Solid Edge part; units mm, degrees
sketch "Sketch1" plane through (0, 0, 0) normal (0, 0, 1) x (1, 0, 0)
  line L0 (-74.7428, -5) -> (-74.7428, -88.7121)
  arc A0 (-70.7682, -93.6058) -> (-74.7428, -88.7121) centre (-69.7428, -88.7121) cw
  arc A1 (-70.7682, -93.6058) -> (70.7677, -93.5993) centre (-0.0157, 244.0613) ccw
  arc A2 (74.7418, -88.7058) -> (70.7677, -93.5994) centre (69.7418, -88.7058) cw
  line L1 (74.7418, -88.7058) -> (74.7418, -5)
  arc A3 (69.7418, 0) -> (74.7418, -5) centre (69.7418, -5) cw
  line L2 (69.7418, 0) -> (65.2418, 0)
  arc A4 (60.2418, -5) -> (65.2418, 0) centre (65.2418, -5) cw
  line L3 (60.2418, -73.162) -> (60.2418, -5)
  arc A5 (56.0999, -78.0878) -> (60.2418, -73.162) centre (55.2418, -73.162) ccw
  arc A6 (-56.1003, -78.0932) -> (56.0999, -78.0878) centre (-0.0157, 244.0613) ccw
  arc A7 (-60.2428, -73.1673) -> (-56.1003, -78.0932) centre (-55.2428, -73.1673) ccw
  line L4 (-60.2428, -73.1673) -> (-60.2428, -5)
  arc A8 (-65.2428, 0) -> (-60.2428, -5) centre (-65.2428, -5) cw
  line L5 (-65.2428, 0) -> (-69.7428, 0)
  arc A9 (-74.7428, -5) -> (-69.7428, 0) centre (-69.7428, -5) cw
extrude "Protrusion1" add sketch "Sketch1" along normal mid plane 12
properties part number "2003-004" material "Plastic"
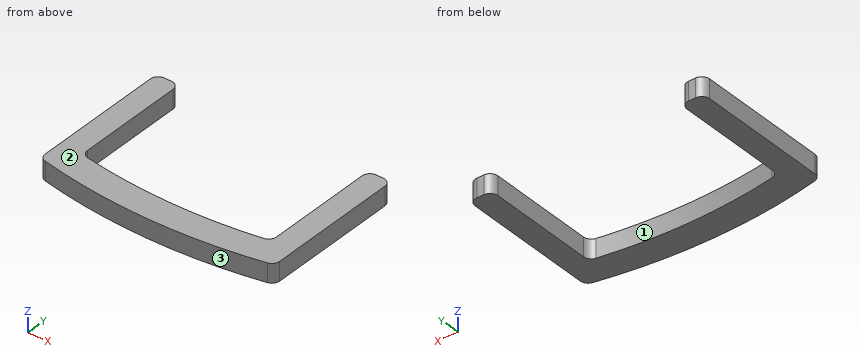
Model file for the job. Use its own axes, mm. Face numbers are marked on the shaded views. Give positions to 0.01 mm unless a question says otherwise; leave off trailing zeros. Write each loop counter-clockwise with the first axis right and the second up, starting at its lowest first coordinate (ties: lowest second). Pieces come first, ordered by that corner, then holes. Notation, with made-up numbers: (-16, 5) - (40, 5) arc R17 cw to (40, 10) - close; hole circle Ø11 at (89, 44). An arc over 180 degrees is marked (long way). One line per question, with ' | ' between items. Start each with the question number.
(1) Wall check: line 1 along X through (y, z) = (-9, 1); line 2 along Y through (x, z) = (3.5, 5.25); line 3 along Y through (x, z) = (55.5, 1.25). Give the ranges that are in metal, low to high. Write a range as from..to.
(2) Pin check, flat tip, straight feed: P1, Ø2, axis at x = -48.5, z = 3.5, coming from the -Y side. Stop position of the tip, or through.
(3) Slice it at A-A on y = -66.5. Write the cut outline in (x, z).
(4) Slice it at B-B on z = 1.5. Write the cut outline in (x, y), plus the area to 3 significant figures.
(5) Slice it at D-D on x = 18.5. Write the cut outline in (y, z), plus the area to 3 significant figures.
(6) Slice it at C-C on x = -20. Write the cut outline in (y, z), plus the area to 3 significant figures.
(7) Two-plate mould, pull along X, no slides. Class the marked faces 1, 2 and 3: +X half, -X half, draft (parallel to the pull), parting line (faces both ways), or undercut.
Results below:
1) line 1: -74.74..-60.24, 60.24..74.74 | line 2: -100.92..-82.92 | line 3: -96.44..-78.19
2) P1: y = -97.66
3) outline: (-74.74, -6) - (-60.24, -6) - (-60.24, 6) - (-74.74, 6) - close; (60.24, -6) - (74.74, -6) - (74.74, 6) - (60.24, 6) - close
4) outline: (-74.74, -88.71) arc R5 ccw to (-70.77, -93.61) arc R345 ccw to (70.77, -93.6) arc R5 ccw to (74.74, -88.71) - (74.74, -5) arc R5 ccw to (69.74, 0) - (65.24, 0) arc R5 ccw to (60.24, -5) - (60.24, -73.16) arc R5 cw to (56.1, -78.09) arc R327 cw to (-56.1, -78.09) arc R5 cw to (-60.24, -73.17) - (-60.24, -5) arc R5 ccw to (-65.24, 0) - (-69.74, 0) arc R5 ccw to (-74.74, -5) - close | area: 4,890 mm^2
5) outline: (-100.44, -6) - (-82.41, -6) - (-82.41, 6) - (-100.44, 6) - close | area: 216 mm^2
6) outline: (-100.36, -6) - (-82.33, -6) - (-82.33, 6) - (-100.36, 6) - close | area: 216 mm^2
7) face 1: undercut | face 2: draft | face 3: parting line
